from build123d import *

# Parameters (mm, degrees)
CROQUIS1_W                = 13
CROQUIS1_H                = 80
SALIENTE_EXTRUIR1_DEPTH   = 4
CROQUIS1_W_2              = 10
SALIENTE_EXTRUIR1_2_DEPTH = 4
SALIENTE_EXTRUIR1_3_DEPTH = 4
CROQUIS2_W                = 13
CROQUIS2_H                = 13
CROQUIS2_W_2              = 10
CROQUIS2_H_2              = 10
SALIENTE_EXTRUIR2_DEPTH   = 10
CROQUIS3_W                = 13
CROQUIS3_H                = 80
CROQUIS3_W_2              = 10
SALIENTE_EXTRUIR3_DEPTH   = 2.2
CROQUIS4_W                = 80
CROQUIS4_H                = 10
CROQUIS4_H_2              = 13
SALIENTE_EXTRUIR4_DEPTH   = 4
CROQUIS5_W                = 80
CROQUIS5_H                = 80
CROQUIS5_W_2              = 75.6
CROQUIS5_H_2              = 75.6
SALIENTE_EXTRUIR5_DEPTH   = 15
CHAFL_N2_SIZE             = 6.4
CHAFL_N3_SIZE             = 6
CHAFL_N4_SIZE             = 2.2
CORTAR_EXTRUIR1_DEPTH     = 0.4
REDONDEO1_R               = 1
CHAFL_N1_SIZE             = 1


with BuildPart() as part:
    # Croquis1 → Saliente-Extruir1 (new body)
    with BuildSketch(Plane(origin=(0, 0, 0), x_dir=(0, 1, 0), z_dir=(0, 0, 1))):
        Rectangle(CROQUIS1_W, CROQUIS1_H)
    extrude(amount=SALIENTE_EXTRUIR1_DEPTH)



with BuildPart() as body_2:
    # Croquis1 → Saliente-Extruir1 2 (new body)
    with BuildSketch(Plane(origin=(0, 0, 0), x_dir=(0, 1, 0), z_dir=(0, 0, 1))):
        with Locations((35, 0)):
            Rectangle(CROQUIS1_W_2, CROQUIS1_H)
    extrude(amount=SALIENTE_EXTRUIR1_2_DEPTH)


with BuildPart() as body_3:
    # Croquis1 → Saliente-Extruir1 3 (new body)
    with BuildSketch(Plane(origin=(0, 0, 0), x_dir=(0, 1, 0), z_dir=(0, 0, 1))):
        with Locations((-35, 0)):
            Rectangle(CROQUIS1_W_2, CROQUIS1_H)
    extrude(amount=SALIENTE_EXTRUIR1_3_DEPTH)


with BuildPart() as part_1:
    add(part.part)

    add(body_2.part)  # Saliente-Extruir2 merges body 2

    add(body_3.part)  # Saliente-Extruir2 merges body 3
    # Croquis2 → Saliente-Extruir2 (add)
    with BuildSketch(Plane.XY.offset(4)):
        Rectangle(CROQUIS2_W, CROQUIS2_H)
        with Locations((-35, 0)):
            Rectangle(CROQUIS2_W_2, CROQUIS2_H)
        with Locations((35, 0)):
            Rectangle(CROQUIS2_W_2, CROQUIS2_H)
        with Locations((0, 35)):
            Rectangle(CROQUIS2_W, CROQUIS2_H_2)
        with Locations((-35, 35)):
            Rectangle(CROQUIS2_W_2, CROQUIS2_H_2)
        with Locations((35, 35)):
            Rectangle(CROQUIS2_W_2, CROQUIS2_H_2)
        with Locations((35, -35)):
            Rectangle(CROQUIS2_W_2, CROQUIS2_H_2)
        with Locations((-35, -35)):
            Rectangle(CROQUIS2_W_2, CROQUIS2_H_2)
        with Locations((0, -35)):
            Rectangle(CROQUIS2_W, CROQUIS2_H_2)
    extrude(amount=SALIENTE_EXTRUIR2_DEPTH)

    # Croquis3 → Saliente-Extruir3 (add)
    with BuildSketch(Plane.XY.offset(14)):
        Rectangle(CROQUIS3_W, CROQUIS3_H)
        with Locations((-35, 0)):
            Rectangle(CROQUIS3_W_2, CROQUIS3_H)
        with Locations((35, 0)):
            Rectangle(CROQUIS3_W_2, CROQUIS3_H)
    extrude(amount=-SALIENTE_EXTRUIR3_DEPTH)

    # Croquis4 → Saliente-Extruir4 (add)
    with BuildSketch(Plane.XY.offset(14)):
        with Locations((0, -35)):
            Rectangle(CROQUIS4_W, CROQUIS4_H)
        Rectangle(CROQUIS4_W, CROQUIS4_H_2)
        with Locations((0, 35)):
            Rectangle(CROQUIS4_W, CROQUIS4_H)
        with Locations((0, 16.5)):
            Rectangle(CROQUIS4_W, CROQUIS4_H)
        with Locations((0, -16.5)):
            Rectangle(CROQUIS4_W, CROQUIS4_H)
    extrude(amount=SALIENTE_EXTRUIR4_DEPTH)

    # Croquis5 → Saliente-Extruir5 (add)
    with BuildSketch(Plane.XY.offset(14)):
        Rectangle(CROQUIS5_W, CROQUIS5_H)
        Rectangle(CROQUIS5_W_2, CROQUIS5_H_2, mode=Mode.SUBTRACT)
    extrude(amount=SALIENTE_EXTRUIR5_DEPTH)

    # Chaflán2
    chafl_n2_edges = [part_1.edges().sort_by_distance(p)[0] for p in [
        (0, -30, 11.8),
        (-35, 6.5, 11.8),
        (-35, -6.5, 11.8),
        (-35, 30, 11.8),
        (-35, -30, 11.8),
        (35, 6.5, 11.8),
        (35, 30, 11.8),
        (35, -6.5, 11.8),
        (35, -30, 11.8),
        (0, 6.5, 11.8),
        (0, -6.5, 11.8),
        (0, 30, 11.8),
    ]]
    chamfer(chafl_n2_edges, length=CHAFL_N2_SIZE)

    # Chaflán3
    chafl_n3_edges = [part_1.edges().sort_by_distance(p)[0] for p in [
        (-6.5, -35, 14),
        (30, -35, 14),
        (6.5, 35, 14),
        (-30, 35, 14),
        (6.5, -35, 14),
        (-6.5, 35, 14),
        (-30, -35, 14),
        (30, 35, 14),
    ]]
    chamfer(chafl_n3_edges, length=CHAFL_N3_SIZE)

    # Chaflán4
    chafl_n4_edges = [part_1.edges().sort_by_distance(p)[0] for p in [
        (30, 16.5, 14),
        (30, -16.5, 14),
        (6.5, -16.5, 14),
        (-6.5, -16.5, 14),
        (-30, -16.5, 14),
        (6.5, 16.5, 14),
        (-30, 16.5, 14),
    ]]
    chamfer(chafl_n4_edges, length=CHAFL_N4_SIZE - 0.0001)  # a hair under: the kernel refuses the full size

    # Croquis6 → Cortar-Extruir1 (cut)
    with BuildSketch(Plane(origin=(-40, 0, 0), x_dir=(0, -1, 0), z_dir=(-1, 0, 0))):
        Polygon((-5, 9.5), (5, 9.5), (3, 19.5), (-3, 19.5), align=None)
    extrude(amount=-CORTAR_EXTRUIR1_DEPTH, mode=Mode.SUBTRACT)

    # Redondeo1
    redondeo1_edges = [part_1.edges().sort_by_distance(p)[0] for p in [
        (-39.8, -3, 19.5),
        (-39.8, -5, 9.5),
        (-39.8, 5, 9.5),
        (-39.8, 3, 19.5),
    ]]
    fillet(redondeo1_edges, radius=REDONDEO1_R)

    # Chaflán1
    chafl_n1_edges = [part_1.edges().sort_by_distance(p)[0] for p in [
        (-40, 40, 14.5),
        (-40, -40, 14.5),
        (40, -40, 14.5),
        (40, 6.5, 2.7),
        (-40, 6.5, 2.7),
        (-30, 6.5, 4.7),
        (-6.5, 6.5, 4.7),
        (6.5, 6.5, 4.7),
        (30, 6.5, 4.7),
        (6.5, -6.5, 4.7),
        (-30, -6.5, 4.7),
        (-40, -6.5, 2.7),
        (40, -6.5, 2.7),
        (-40, -18.25, 11.8),
        (30, 30, 4.7),
        (-6.5, 30, 4.7),
        (-30, 30, 4.7),
        (-40, 30, 2.7),
        (40, 30, 2.7),
        (-40, 18.25, 11.8),
        (40, -30, 2.7),
        (-40, -30, 2.7),
        (-30, -30, 4.7),
        (6.5, -30, 4.7),
        (30, -30, 4.7),
        (40, 18.25, 11.8),
        (40, -18.25, 11.8),
        (-40, -9.7, 8.6),
        (-40, 26.8, 8.6),
        (-40, 9.7, 8.6),
        (-40, -26.8, 8.6),
        (40, 9.7, 8.6),
        (40, 26.8, 8.6),
        (40, -9.7, 8.6),
        (40, -26.8, 8.6),
        (30, 40, 6),
        (30, -40, 6),
        (-30, 40, 6),
        (-30, -40, 6),
        (6.5, 40, 6),
        (-6.5, -40, 6),
        (6.5, -40, 6),
        (-6.5, 40, 6),
        (40, 40, 14.5),
    ]]
    chamfer(chafl_n1_edges, length=CHAFL_N1_SIZE)


solid = part_1.part
Geometry: final body of the model. Coordinates: model frame, mm. A direction names the side the tool comes from. Round coordinates to 2 decimals unless told otherwise and drop trailing zeros. Order: outer loops, then holes, each group sorted by start corner. A loop starts at its lowest first (then second) coordinate and runs counter-clockwise, first axis right, second up.
Q1. Mould query, pull axis Z, two halves, no side actions, for faces 4 (the face through (40, -1, 18)), 5 (the face through (-39.493, 27.1, 8.998)), 6 (the face through (18, -35, 4)), 7 (the face through (-27, 35, 11)). Classes: released by +Z, released by -Z, zero draft, split by the parting line, or undercut.
Result sheet:
face 4: zero draft
face 5: released by -Z
face 6: undercut
face 7: undercut
Q2. Section D-D, the plane x = -10.5. Give the number of separate pieces and of enclosed holes in the cut face, and give its area (3 significant figures).
Result sheet:
separate pieces: 8
enclosed holes: 0
area: 432 mm2
Q3. Section A-A, the plane z = 20.5. Output: boundary loops of the cut face in (x, y), and give its area (3 significant figures).
Result sheet:
outline: (-40, -39) - (-39, -40) - (39, -40) - (40, -39) - (40, 39) - (39, 40) - (-39, 40) - (-40, 39) - close; hole (-37.8, -37.8) - (37.8, -37.8) - (37.8, 37.8) - (-37.8, 37.8) - close
area: 683 mm2
Q4. Access query for faces 1 (the face through (-1, 37.8, 23)), 2 (the face through (-1, 6.5, 2)), 3 (the face through (28.9, 16.4, 12.9)). Directions: +Z, -Z, +X, -X, +Y, -Y. A direction counts if a zero-diameter tool reaches every point of the face in a straight line with its end or side. Return the directions, or none.
Result sheet:
face 1: +Z
face 2: -Z, +X, -X
face 3: -Z
Q5. Section C-C, the plane y = -25. Output: boundary loops of the cut face in (x, z), and give its area (3 significant figures).
Result sheet:
outline: (-40, 11.81) - (-39, 10.4) - (-30, 10.4) - (-30, 14) - (-37.8, 14) - (-37.8, 29) - (-40, 29) - close; (-6.5, 10.4) - (6.5, 10.4) - (6.5, 14) - (-6.5, 14) - close; (30, 10.4) - (39, 10.4) - (40, 11.81) - (40, 29) - (37.8, 29) - (37.8, 14) - (30, 14) - close
area: 183 mm2
Q6. Material intervals for probe 1 along Y at (x, z) = (-21.5, 3.5); probe 2 along Y at (x, z) = (-35.5, 19.25), sorted ascending.
Result sheet:
probe 1: y = -40 to -30, -6.5 to 6.5, 30 to 40
probe 2: y = -40 to -37.8, 37.8 to 40
Q7. Pin query (flat end, axial travel): pin 1 (5 mm diameter, centred on x = 15, y = 17.5, fed in from -Z); pin 2 (8.5 mm diameter, centred on x = 32, y = 27.5, fed in from +Z); pin 3 (8 mm diameter, centred on y = -16.5, z = 11, fed in from -X); pin 4 (7 mm diameter, centred on x = 32.5, y = -19, fed in from -Z). Return the tip coordinate at first contact, or that it passes through.
Result sheet:
pin 1: stops at z = 14
pin 2: stops at z = 18
pin 3: stops at x = -40
pin 4: stops at z = 11.8
